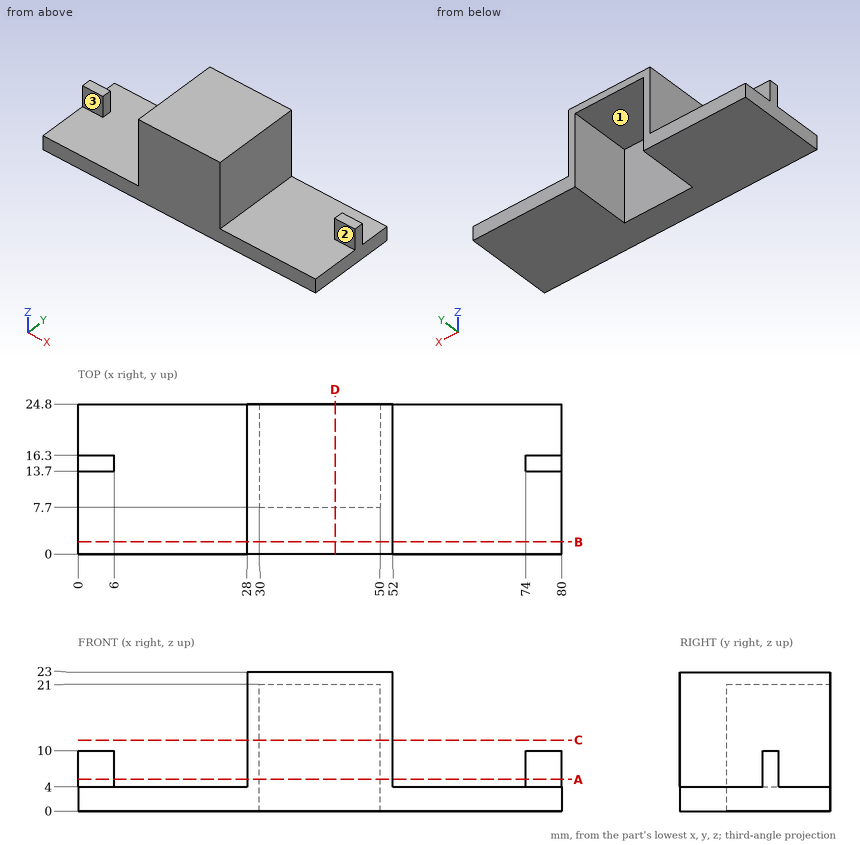
Part print with two shaded views. Sizes in mm from the minimum x, y, z corner. A direction names the side the tool comes from. Round coordinates to 2 decimals unless told otherwise and drop trailing zeros. Order: outer loops, then holes, each group sorted by start corner. A loop starts at its lowest first (then second) coordinate and runs counter-clockwise, first axis right, second up. Notation, with made-up numbers: M 38.5,69.5 L 60.5,69.5 A19 cw 60.5,85.5 Z; hole C 85.5,74 d7. An arc over 180 degrees is marked long. Put each result on its own line as item: value. Start each with the question number.
1. Tool access for the marked faces 1, 2 and 3: list every direction of +Z, -Z, +X, -X, +Y, -Y with a clear straight run to the whole face (end or side of a thin tool).
2. Slice it at B-B on y = 2. List the corners of the cut face in (x, z).
3. Drill centre lines: probe 1 along X at (y, z) = (14, 7.75); probe 2 along X at (y, z) = (16.75, 12.5); probe 3 along X at (y, z) = (14.75, 3.25). Where is each one in solid material? Low to high. Write a range as [from, to].
4. Drop flat-ended pins along their axis: pin 1 (1 mm diameter, centred on x = 17.5, y = 18, fed in from +Z); pin 2 (1.8 mm diameter, centred on x = 77, z = 7.5, fed in from -Y); pin 3 (2 mm diameter, centred on x = 77.5, y = 15.5, fed in from +Z). Give the stop position or say it passes through.
5. Slice it at A-A on z = 5.25. List the corners of the cut face in (x, y), then the cut area to 3 significant figures.
6. Slice it at C-C on z = 11.75. List the corners of the cut face in (x, y), then the cut area to 3 significant figures.
7. Slice it at D-D on x = 42.5. List the corners of the cut face in (y, z).
Findings:
1. face 1: -Z, +Y
1. face 2: +Z, +X, -Y
1. face 3: +Z, -X, -Y
2. outline: M 0,0 L 80,0 L 80,4 L 52,4 L 52,23 L 28,23 L 28,4 L 0,4 Z
3. probe 1: [0, 6], [28, 30], [50, 52], [74, 80]
3. probe 2: [28, 30], [50, 52]
3. probe 3: [0, 30], [50, 80]
4. pin 1: z = 4
4. pin 2: y = 13.7
4. pin 3: z = 10
5. outline: M 0,13.7 L 6,13.7 L 6,16.3 L 0,16.3 Z; M 28,0 L 52,0 L 52,24.8 L 50,24.8 L 50,7.7 L 30,7.7 L 30,24.8 L 28,24.8 Z; M 74,13.7 L 80,13.7 L 80,16.3 L 74,16.3 Z
5. area: 284 mm2
6. outline: M 28,0 L 52,0 L 52,24.8 L 50,24.8 L 50,7.7 L 30,7.7 L 30,24.8 L 28,24.8 Z
6. area: 253 mm2
7. outline: M 0,0 L 7.7,0 L 7.7,21 L 24.8,21 L 24.8,23 L 0,23 Z
